Could you check a few things on this model? Use its own coordinates, in mm. A direction names the side the tool comes from. Round coordinates to 2 decimals unless told otherwise and drop trailing zeros. Write each loop counter-clockwise with the first axis right and the second up, starting at its lowest first coordinate (ties: lowest second). Pieces come first, ordered by that corner, then holes. Notation, with made-up numbers: (-28.5, -28.5) -> (30.5, -28.5) arc R6 cw to (30.5, -18.5) -> close; hole circle Ø1 at (67.5, -16.75). An arc over 180 degrees is marked (long way). Return JSON: item names as keys, results as strings.
from build123d import *

# Parameters (mm, degrees)
SKETCH1_W           = 60
SKETCH1_H           = 40
BOSS_EXTRUDE1_DEPTH = 10
SKETCH2_W           = 10
SKETCH2_H           = 40
BOSS_EXTRUDE2_DEPTH = 30
SKETCH3_W           = 40
SKETCH3_H           = 10
BOSS_EXTRUDE3_DEPTH = 74
SKETCH4_R           = 6.1
SKETCH4_R_2         = 3.15
CUT_EXTRUDE1_DEPTH  = 74
SKETCH5_R           = 3
CUT_EXTRUDE2_DEPTH  = 74
SKETCH6_R           = 3.5
CUT_EXTRUDE3_DEPTH  = 3
SKETCH7_R           = 6.5
CUT_EXTRUDE4_DEPTH  = 5
M3_TAPPED_HOLE1_D   = 2.5
CIRPATTERN1_COUNT   = 4
SKETCH10_W          = 60
SKETCH10_H          = 5
BOSS_EXTRUDE4_DEPTH = 3


with BuildPart() as part:
    # Sketch1 → Boss-Extrude1 (new body)
    with BuildSketch(Plane(origin=(0, 0, 0), x_dir=(1, 0, 0), z_dir=(0, 1, 0))):
        Rectangle(SKETCH1_W, SKETCH1_H)
    extrude(amount=BOSS_EXTRUDE1_DEPTH)

    # Sketch2 → Boss-Extrude2 (add)
    with BuildSketch(Plane(origin=(0, 10, 0), x_dir=(1, 0, 0), z_dir=(0, 1, 0))):
        with Locations((-25, 0)):
            Rectangle(SKETCH2_W, SKETCH2_H)
    extrude(amount=BOSS_EXTRUDE2_DEPTH)

    # Sketch3 → Boss-Extrude3 (add)
    with BuildSketch(Plane.ZY.offset(30)):
        with Locations((0, 35)):
            Rectangle(SKETCH3_W, SKETCH3_H)
    extrude(amount=BOSS_EXTRUDE3_DEPTH)

    # Sketch4 → Cut-Extrude1 (cut)
    with BuildSketch(Plane.XZ.offset(-30)):
        with Locations(Location((-53, 0, 0), (0, 0, 270))):
            Circle(SKETCH4_R)
        with Locations(Location((-71, 0, 0), (0, 0, 270))):
            Circle(SKETCH4_R_2)
        with Locations(Location((-89, 0, 0), (0, 0, 270))):
            Circle(SKETCH4_R_2)
    extrude(amount=-CUT_EXTRUDE1_DEPTH, mode=Mode.SUBTRACT)

    # Sketch5 → Cut-Extrude2 (cut)
    with BuildSketch(Plane.XZ):
        with Locations(Location((-11.5, 8.5, 0), (0, 0, 270))):
            Circle(SKETCH5_R)
        with Locations(Location((-11.5, -8.5, 0), (0, 0, 270))):
            Circle(SKETCH5_R)
        with Locations(Location((3.5, 8.5, 0), (0, 0, 270))):
            Circle(SKETCH5_R)
        with Locations(Location((3.5, -8.5, 0), (0, 0, 270))):
            Circle(SKETCH5_R)
    extrude(amount=-CUT_EXTRUDE2_DEPTH, mode=Mode.SUBTRACT)

    # Sketch6 → Cut-Extrude3 (cut)
    with BuildSketch(Plane.XZ.offset(-30)):
        with Locations(Location((-89, 0, 0), (0, 0, 270))):
            Circle(SKETCH6_R)
        with Locations(Location((-71, 0, 0), (0, 0, 270))):
            Circle(SKETCH6_R)
    extrude(amount=-CUT_EXTRUDE3_DEPTH, mode=Mode.SUBTRACT)

    # Sketch7 → Cut-Extrude4 (cut)
    with BuildSketch(Plane.XZ.offset(-30)):
        with Locations(Location((-53, 0, 0), (0, 0, 270))):
            Circle(SKETCH7_R)
    extrude(amount=-CUT_EXTRUDE4_DEPTH, mode=Mode.SUBTRACT)

    # M3 Tapped Hole1 (through all)
    with Locations(Plane(origin=(0, 40, 0), x_dir=(1, 0, 0), z_dir=(0, 1, 0))):
        with Locations((-53, 12.5)):
            m3_tapped_hole1 = Hole(M3_TAPPED_HOLE1_D / 2)

    # CirPattern1: M3 Tapped Hole1 ×4 about axis
    cirpattern1_axis = Axis((-53, 0, 0), (0, 1, 0))
    for i in range(1, CIRPATTERN1_COUNT):
        add(m3_tapped_hole1.rotate(cirpattern1_axis, i * 360 / CIRPATTERN1_COUNT), mode=Mode.SUBTRACT)

    # Sketch10 → Boss-Extrude4 (add)
    with BuildSketch(Plane.XZ):
        with Locations((0, -17.5)):
            Rectangle(SKETCH10_W, SKETCH10_H)
    extrude(amount=BOSS_EXTRUDE4_DEPTH)


solid = part.part
1) Will these pins go through, and if not, where does the flat tip stop? pin 1 Ø9.5 at (x, z) = (3.5, -8.5) entering from +Y; pin 2 Ø10 at (x, z) = (-64.5, 9.5) entering from -Y; pin 3 Ø8 at (x, z) = (-11.5, 8.5) entering from -Y.
Return value:
{"pin 1": "y = 10", "pin 2": "y = 30", "pin 3": "y = 0"}
2) If I drill on probe 1 along X at (y, z) = (32.35, 0); probe 2 along X at (y, z) = (37.35, 0); probe 3 along X at (y, z) = (9, -6.5), over which ranges is the centre line in solid material (lowest first)? Write a range as [from, to].
Return value:
{"probe 1": "[-104, -92.5], [-85.5, -74.5], [-67.5, -66.75], [-64.25, -59.5], [-46.5, -41.75], [-39.25, -20]", "probe 2": "[-104, -92.15], [-85.85, -74.15], [-67.85, -66.75], [-64.25, -59.1], [-46.9, -41.75], [-39.25, -20]", "probe 3": "[-30, -13.74], [-9.26, 1.26], [5.74, 30]"}
3) I want a section at A-A, the plane x = -40.5. Please give me the cut outline in (y, z).
Return value:
{"outline": "(30, -20) -> (40, -20) -> (40, -1.25) -> (30, -1.25) -> close; (30, 1.25) -> (40, 1.25) -> (40, 20) -> (30, 20) -> close"}
4) For faces 1 (the face through (-20, 25, 0)), 2 (the face through (-59.345, 32.465, 1.409)), 3 (the face through (-66, 30, -5)), which set-ups out of +Z, -Z, +X, -X, +Y, -Y let a thin tool reach every point of the face, with its end or its side?
Return value:
{"face 1": "+Z, -Z, +X, +Y", "face 2": "-Y", "face 3": "+Z, -Z, -X, -Y"}
5) Thinking about a two-plate mould opening in Z: for faces 4 (the face through (-41.609, 34.93, -0.577)), 5 (the face through (-74.417, 31.479, 0.759)), 6 (the face through (5, 10, 0)), which applies, pulls with the +Z half, pulls with the -Z half, needs draft (parallel to the pull), parting line crosses it, or undercut?
Return value:
{"face 4": "undercut", "face 5": "undercut", "face 6": "needs draft"}
6) I want a section at D-D, the plane x = 21. Please give me the cut outline in (y, z), and give its area (3 significant figures).
Return value:
{"outline": "(-3, -20) -> (10, -20) -> (10, 20) -> (0, 20) -> (0, -15) -> (-3, -15) -> close", "area": "415 mm²"}
7) I want a section at B-B, the plane z = -8.5. Please give me the cut outline in (x, y).
Return value:
{"outline": "(-104, 30) -> (-30, 30) -> (-30, 0) -> (-14.5, 0) -> (-14.5, 10) -> (-20, 10) -> (-20, 40) -> (-104, 40) -> close; (-8.5, 0) -> (0.5, 0) -> (0.5, 10) -> (-8.5, 10) -> close; (6.5, 0) -> (30, 0) -> (30, 10) -> (6.5, 10) -> close"}
8) I want a section at C-C, the plane x = 3.5. Please give me the cut outline in (y, z), and give its area (3 significant figures).
Return value:
{"outline": "(-3, -20) -> (10, -20) -> (10, -11.5) -> (0, -11.5) -> (0, -15) -> (-3, -15) -> close; (0, -5.5) -> (10, -5.5) -> (10, 5.5) -> (0, 5.5) -> close; (0, 11.5) -> (10, 11.5) -> (10, 20) -> (0, 20) -> close", "area": "295 mm²"}
